```python
from build123d import *

# Parameters (mm, degrees)
F0_W     = 40
F0_H     = 35
F0_R     = 10.25
F0_R_2   = 4
F0_R_3   = 2.25
F0_R_4   = 1.5
F0_R_5   = 4.25
F1_DEPTH = 10
F2_DEPTH = 6
F3_DEPTH = 3
F5_DEPTH = 3
F6_R     = 5


with BuildPart() as f1:
    # F0 (on Front) → F1 (new body)
    with BuildSketch(Plane.XZ):
        with Locations((0, 5.5)):
            Rectangle(F0_W, F0_H)
        Circle(F0_R, mode=Mode.SUBTRACT)
        with Locations((-12.5, 13)):
            Circle(F0_R_2, mode=Mode.SUBTRACT)
        with Locations((12.5, 13)):
            Circle(F0_R_2, mode=Mode.SUBTRACT)
        with Locations((-12.5, 13)):
            Circle(F0_R_2)
        with Locations((-12.5, 13)):
            Circle(F0_R_3, mode=Mode.SUBTRACT)
        with Locations((12.5, 13)):
            Circle(F0_R_2)
        with Locations((12.5, 13)):
            Circle(F0_R_3, mode=Mode.SUBTRACT)
        Circle(F0_R)
        with Locations((-5.629165, -3.25)):
            Circle(F0_R_4, mode=Mode.SUBTRACT)
        Circle(F0_R_5, mode=Mode.SUBTRACT)
        with Locations((5.629165, -3.25)):
            Circle(F0_R_4, mode=Mode.SUBTRACT)
        with Locations((0, 6.5)):
            Circle(F0_R_4, mode=Mode.SUBTRACT)
    extrude(amount=-F1_DEPTH)

    # F0 (on Front) → F2 (cut)
    with BuildSketch(Plane.XZ):
        with Locations((12.5, 13)):
            Circle(F0_R_2)
        with Locations((12.5, 13)):
            Circle(F0_R_3, mode=Mode.SUBTRACT)
        with Locations((-12.5, 13)):
            Circle(F0_R_2)
        with Locations((-12.5, 13)):
            Circle(F0_R_3, mode=Mode.SUBTRACT)
    extrude(amount=-F2_DEPTH, mode=Mode.SUBTRACT)

    # F0 (on Front) → F3 (cut)
    with BuildSketch(Plane.XZ):
        Circle(F0_R)
        with Locations((-5.629165, -3.25)):
            Circle(F0_R_4, mode=Mode.SUBTRACT)
        Circle(F0_R_5, mode=Mode.SUBTRACT)
        with Locations((5.629165, -3.25)):
            Circle(F0_R_4, mode=Mode.SUBTRACT)
        with Locations((0, 6.5)):
            Circle(F0_R_4, mode=Mode.SUBTRACT)
    extrude(amount=-F3_DEPTH, mode=Mode.SUBTRACT)

    # F4 (on face) → F5 (cut)
    with BuildSketch(Plane(origin=(0, 10, 0), x_dir=(-1, 0, 0), z_dir=(0, 1, 0))):
        with BuildLine():
            Line((1.732051, 9.5), (-1.732051, 9.5))
            Line((-1.732051, 9.5), (-3.464102, 6.5))
            Line((-3.464102, 6.5), (-1.732051, 3.5))
            Line((-1.732051, 3.5), (-2.165064, 2.75))
            ThreePointArc((-2.165064, 2.75), (0, 3.5), (2.165064, 2.75))
            Line((2.165064, 2.75), (1.732051, 3.5))
            Line((1.732051, 3.5), (3.464102, 6.5))
            Line((3.464102, 6.5), (1.732051, 9.5))
        make_face()
        with BuildLine():
            Line((-3.464102, 0.5), (-2.165064, 2.75))
            ThreePointArc((-2.165064, 2.75), (-3.031089, 1.75), (-3.464102, 0.5))
        make_face()
        with BuildLine():
            ThreePointArc((3.464102, 0.5), (3.031089, 1.75), (2.165064, 2.75))
            Line((2.165064, 2.75), (3.464102, 0.5))
        make_face()
        with BuildLine():
            ThreePointArc((-1.299038, -3.25), (-3.031089, -1.75), (-3.464102, 0.5))
            Line((-3.464102, 0.5), (-3.897114, -0.25))
            Line((-3.897114, -0.25), (-7.361216, -0.25))
            Line((-7.361216, -0.25), (-9.093267, -3.25))
            Line((-9.093267, -3.25), (-7.361216, -6.25))
            Line((-7.361216, -6.25), (-3.897114, -6.25))
            Line((-3.897114, -6.25), (-2.165064, -3.25))
            Line((-2.165064, -3.25), (-1.299038, -3.25))
        make_face()
        with BuildLine():
            Line((3.897114, -0.25), (3.464102, 0.5))
            ThreePointArc((3.464102, 0.5), (3.491014, 0.250644), (3.5, 0))
            ThreePointArc((3.5, 0), (2.897985, -1.962571), (1.299038, -3.25))
            Line((1.299038, -3.25), (2.165064, -3.25))
            Line((2.165064, -3.25), (3.897114, -6.25))
            Line((3.897114, -6.25), (7.361216, -6.25))
            Line((7.361216, -6.25), (9.093267, -3.25))
            Line((9.093267, -3.25), (7.361216, -0.25))
            Line((7.361216, -0.25), (3.897114, -0.25))
        make_face()
        with BuildLine():
            Line((1.299038, -3.25), (-1.299038, -3.25))
            ThreePointArc((-1.299038, -3.25), (0, -3.5), (1.299038, -3.25))
        make_face()
    extrude(amount=-F5_DEPTH, mode=Mode.SUBTRACT)

    # F6
    f6_edges = [f1.edges().sort_by_distance(p)[0] for p in [
        (-20, 5, 23),
        (20, 5, 23),
        (20, 5, -12),
        (-20, 5, -12),
    ]]
    fillet(f6_edges, radius=F6_R)


solid = f1.part
```
Build history of the part. All positions in model axes, mm. A direction names the side the tool comes from. Give positions to 0.01 mm unless a question says otherwise; leave off trailing zeros. Loops run counter-clockwise (first coordinate to the right, second up) from the corner with the lowest first, then second, coordinate; pieces in that order, holes last.
1) Band-saw the part on C-C on x = 0. List the corners of the cut face in (y, z), then the cut area to 3 significant figures.
Values follow:
outline: (0, -12) - (10, -12) - (10, -4.25) - (3, -4.25) - (3, -10.25) - (0, -10.25) - close; (0, 10.25) - (3, 10.25) - (3, 8) - (7, 8) - (7, 9.5) - (10, 9.5) - (10, 23) - (0, 23) - close; (3, 4.25) - (7, 4.25) - (7, 5) - (3, 5) - close
area: 201 mm2
2) 3-axis set-ups, long thin cutter, end or side, ignore diameter. For faces 4 (the face through (-2.222, 1.479, -10.006)), 5 (the face through (0, 5, 23)), 6 (the face through (-2.6, 8.5, 8)): which of +Z, -Z, +X, -X, +Y, -Y reach the whole face in a straight line?
Values follow:
face 4: -Y
face 5: +Z, +X, -X, +Y, -Y
face 6: +Y
3) Band-saw the part on D-D on z = 6. List the corners of the cut face in (x, y).
Values follow:
outline: (-20, 0) - (-8.31, 0) - (-8.31, 3) - (-1.41, 3) - (-1.41, 7) - (-3.18, 7) - (-3.18, 10) - (-20, 10) - close; (1.41, 3) - (8.31, 3) - (8.31, 0) - (20, 0) - (20, 10) - (3.18, 10) - (3.18, 7) - (1.41, 7) - close
4) Band-saw the part on B-B on y = 2.25. List the corners of the cut face in (x, z).
Values follow:
outline: (-20, -7) arc R5 ccw to (-15, -12) - (15, -12) arc R5 ccw to (20, -7) - (20, 18) arc R5 ccw to (15, 23) - (-15, 23) arc R5 ccw to (-20, 18) - close; hole circle Ø8 at (-12.5, 13); hole circle Ø20.5 at (0, 0); hole circle Ø8 at (12.5, 13)
5) Drop flat-ended pins along their axis: P1, Ø4, axis at x = 0, z = 6.5, coming from the -Y side; P2, Ø1.8, axis at x = -7, z = -3, coming from the +Y side. Give the stop position or say it passes through.
Values follow:
P1: stops at y = 3
P2: stops at y = 7
6) Probe line 1 along Z through (x, y) = (0, 3.5); line 2 along Z through (x, y) = (12.5, 8.15); line 3 along X through (y, z) = (5.5, -1). List the from-to ranges inside material, lowest first.
Values follow:
line 1: z = -12 to -4.25, 4.25 to 5, 8 to 23
line 2: z = -12 to 10.75, 15.25 to 23
line 3: x = -20 to -4.13, 4.13 to 20
7) Band-saw the part on A-A on x = -12.5. List the corners of the cut face in (y, z), then the cut area to 3 significant figures.
Values follow:
outline: (0, -12) - (10, -12) - (10, 10.75) - (6, 10.75) - (6, 9) - (0, 9) - close; (0, 17) - (6, 17) - (6, 15.25) - (10, 15.25) - (10, 23) - (0, 23) - close
area: 284 mm2
8) Two-plate mould, pull along Z, no slides. Class faces 1 (the face through (2.695, 8.521, 5.169)), 2 (the face through (-19, 5, 21)), 3 (the face through (20, 5, 5)): released by +Z, released by -Z, zero draft, split by the parting line, or undercut.
Values follow:
face 1: undercut
face 2: released by +Z
face 3: zero draft
